```python
from build123d import *

# Parameters (mm, degrees)
F2_DEPTH = 10


with BuildPart() as f2:
    # F1 (on Right) → F2 (new body)
    with BuildSketch(Plane.YZ):
        Polygon((-4.9547005384, 0), (-3.8, 2), (-5.3601791831, 1.8848744112), (-5.5, 3.7797227268), (0, 4.18556761), (0, 6), (-6.9916076098, 6), (-6.9916076098, 0), align=None)
        Polygon((-6.9916076098, 6.3426704399), (-6.9916076098, 6), (0, 6.3426704399), align=None)
        Polygon((0, 6.3426704399), (-6.9916076098, 6), (0, 6), align=None)
        Polygon((0, 6), (0, 4.18556761), (5.5, 3.7797227268), (5.3601791831, 1.8848744112), (3.8, 2), (4.9547005384, 0), (6.9916076098, 0), (6.9916076098, 6), align=None)
        Polygon((6.9916076098, 6), (0, 6.3426704399), (0, 6), align=None)
        Polygon((6.9916076098, 6.3426704399), (0, 6.3426704399), (6.9916076098, 6), align=None)
    extrude(amount=F2_DEPTH)


solid = f2.part
```
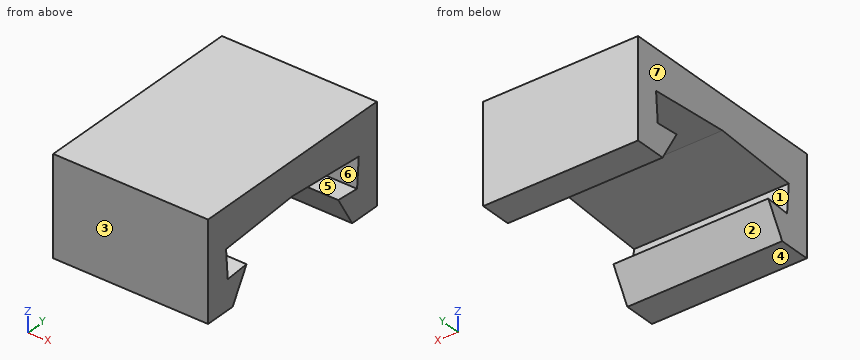
CAD build for the part. Positions are in the model's coordinates, mm. Face numbers are marked on the shaded views. A direction names the side the tool comes from. Coordinates: 2 decimals unless noted, no trailing zeros. Loops run counter-clockwise (first coordinate to the right, second up) from the corner with the lowest first, then second, coordinate; pieces in that order, holes last. Notation, with made-up numbers: (-3.75, 15) - (30.25, 15) arc R19 ccw to (30.25, 40) - close; hole circle Ø6 at (21, 9). An arc over 180 degrees is marked (long way). Use CSV: the item, a comma, the result in double quotes. Start each with the question number.
Q1. Cut at B-B, the plane z = 1. List the corners of the cut face in (x, y), then the cut area to 3 significant figures.
Q2. Drop a flat-ended pin along its axis: P1, Ø4, axis at x = 5.5, y = 0.5, coming from the -Z side. Give the stop position or say it passes through.
Q3. Cut at C-C, the plane z = 3.5. List the corners of the cut face in (x, y), then the cut area to 3 significant figures.
Q4. Cut at D-D, the plane y = -1. List the corners of the cut face in (x, z).
Q5. Probe probe 1 along Y at (x, z) = (2, 1.5); probe 2 along Y at (x, z) = (9.5, 2.5); probe 3 along Z at (x, y) = (1.5, 5). List the from-to ranges inside material, lowest first. Write a range as from..to.
Q6. Two-plate mould, pull along Z, no slides. Class the marked faces 4, 5, 6 and 7: +Z half, -Z half, draft (parallel to the pull), parting line (faces both ways), or undercut.
Q7. Cut at A-A, the plane x = 7. List the corners of the cut face in (y, z), then the cut area to 3 significant figures.
Q8. 3-axis set-ups, long thin cutter, end or side, ignore diameter. For the marked faces 1, 2 and 3: which of +Z, -Z, +X, -X, +Y, -Y reach the whole face in a straight line?
Here are the results:
1,outline,"(0, -6.99) - (10, -6.99) - (10, -4.38) - (0, -4.38) - close; (0, 4.38) - (10, 4.38) - (10, 6.99) - (0, 6.99) - close"
1,area,"52.3 mm2"
2,P1,"z = 4"
3,outline,"(0, -6.99) - (10, -6.99) - (10, -5.48) - (0, -5.48) - close; (0, 5.48) - (10, 5.48) - (10, 6.99) - (0, 6.99) - close"
3,area,"30.2 mm2"
4,outline,"(0, 4.11) - (10, 4.11) - (10, 6.34) - (0, 6.34) - close"
5,probe 1,"-6.99..-4.09, 4.09..6.99"
5,probe 2,"-6.99..-5.41, 5.41..6.99"
5,probe 3,"0..1.91, 3.82..6.34"
6,face 4,"-Z half"
6,face 5,"undercut"
6,face 6,"undercut"
6,face 7,"draft"
7,outline,"(-6.99, 0) - (-4.95, 0) - (-3.8, 2) - (-5.36, 1.88) - (-5.5, 3.78) - (0, 4.19) - (5.5, 3.78) - (5.36, 1.88) - (3.8, 2) - (4.95, 0) - (6.99, 0) - (6.99, 6.34) - (-6.99, 6.34) - close"
7,area,"49.4 mm2"
8,face 1,"+X, -X"
8,face 2,"-Z, +X, -X"
8,face 3,"+Z, -Z, +X, -X, -Y"
